Study the drawing (mm; zero at the part's minimum x, y, z) and answer. A direction names the side the tool comes from. Give positions to 0.01 mm unless a question says otherwise; leave off trailing zeros. Loops run counter-clockwise (first coordinate to the right, second up) from the corner with the lowest first, then second, coordinate; pieces in that order, holes last. Notation, with made-up numbers: M 8.5,40.25 L 67.5,40.25 A19 ccw 67.5,74.25 Z; hole C -29,50.25 d11. An arc over 180 degrees is marked long. Use one line per item in the form item = value. Start each with the question number.
1. The mould has two halves that part along X. Classify the marked faces 1, 2 and 3: released by +X, released by -X, zero draft, split by the parting line, or undercut.
2. Each of these flat-tipped pins is pushed along its axis until it touches: pin 1 Ø3 at (y, z) = (28.5, 8.5) entering from +X; pin 2 Ø4 at (x, z) = (16.5, 7) entering from +Y; pin 3 Ø3 at (y, z) = (33, 1.5) entering from -X; pin 4 Ø10 at (x, y) = (12.5, 6) entering from +Z. Where does it stop, or does it pass through?
3. The part is cut by section A-A (y = 20). Write down the section's boundary in (x, z), and give its area (3 significant figures).
4. The part is cut by section B-B (z = 1.25). Write down the section's boundary in (x, y).
5. The part is cut by section D-D (x = 35). Write down the section's boundary in (y, z).
6. For the marked faces 4 and 5, determine the directions among +Z, -Z, +X, -X, +Y, -Y from which every point of the face is accessible in a straight line to the end or side of a thin tool.
7. Straight lines are drawn through the part: line 1 (X direction, y = 12.5, z = 7); line 2 (X direction, y = 26, z = 3.5); line 3 (Y direction, x = 22, z = 2.75). For each, find the intervals that lie inside material, in ascending order. Write a range as from..to.
8. The part is cut by section C-C (y = 33.5). Write down the section's boundary in (x, z), and give its area (3 significant figures).
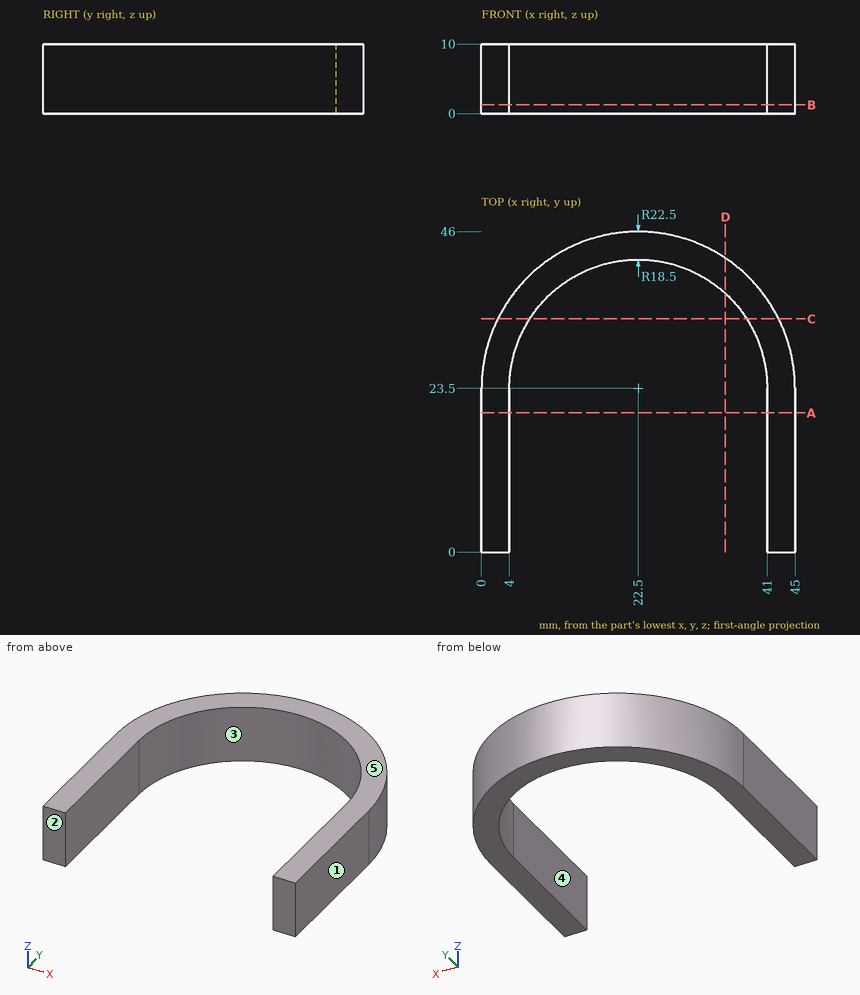
Derived:
q1.face_1 = released by +X
q1.face_2 = zero draft
q1.face_3 = undercut
q2.pin_1 = 44.73
q2.pin_2 = 45.64
q2.pin_3 = 1.47
q2.pin_4 = through
q3.outline = M 0,0 L 4,0 L 4,10 L 0,10 Z; M 41,0 L 45,0 L 45,10 L 41,10 Z
q3.area = 80.0 mm2
q4.outline = M 0,0 L 4,0 L 4,23.5 A18.5 cw 41,23.5 L 41,0 L 45,0 L 45,23.5 A22.5 ccw 0,23.5 Z
q5.outline = M 37.14,0 L 42.21,0 L 42.21,10 L 37.14,10 Z
q6.face_4 = +Z, -Z, -Y
q6.face_5 = +Z, +X, -X, +Y, -Y
q7.line_1 = 0..4, 41..45
q7.line_2 = 0.14..4.17, 40.83..44.86
q7.line_3 = 41.99..45.99
q8.outline = M 2.34,0 L 6.94,0 L 6.94,10 L 2.34,10 Z; M 38.06,0 L 42.66,0 L 42.66,10 L 38.06,10 Z
q8.area = 91.8 mm2
